The model under review builds one solid part; all positions refer to its coordinate system, in mm. Round coordinates to 2 decimals unless told otherwise and drop trailing zeros. Loops run counter-clockwise (first coordinate to the right, second up) from the corner with the lowest first, then second, coordinate; pieces in that order, holes last. Notation, with made-up numbers: (79, -13.5) - (133, -13.5) arc R31 ccw to (133, 19.5) - close; hole circle Ø2 at (52.5, -11.75). An arc over 180 degrees is marked (long way). Answer as CSV lines item,"result".
from build123d import *

# Parameters (mm, degrees)
SKETCH1_R           = 4
BOSS_EXTRUDE1_DEPTH = 50
CHAMFER1_SIZE       = 0.25
CHAMFER2_SIZE       = 0.25
CUT_EXTRUDE2_DEPTH  = 51.318982502


with BuildPart() as part:
    # Sketch1 → Boss-Extrude1 (new body)
    with BuildSketch(Plane.XY):
        Circle(SKETCH1_R)
    extrude(amount=BOSS_EXTRUDE1_DEPTH)

    # Chamfer1
    chamfer1_edges = [part.edges().sort_by_distance(p)[0] for p in [
        (-4, 0, 50),
    ]]
    chamfer(chamfer1_edges, length=CHAMFER1_SIZE)

    # Chamfer2
    chamfer2_edges = [part.edges().sort_by_distance(p)[0] for p in [
        (-4, 0, 0),
    ]]
    chamfer(chamfer2_edges, length=CHAMFER2_SIZE)

    # Sketch4 → Cut-Extrude2 (cut, through all)
    with BuildSketch(Plane.XY.offset(50)):
        with BuildLine():
            Line((-1.5, 3.708099244), (1.5, 3.708099244))
            ThreePointArc((1.5, 3.708099244), (0, 4), (-1.5, 3.708099244))
        make_face()
    extrude(amount=-CUT_EXTRUDE2_DEPTH, mode=Mode.SUBTRACT)


solid = part.part
1. Wall thickness on probe 1 along Y at (x, z) = (1.75, 31.5); probe 2 along Y at (x, z) = (1.5, 14); probe 3 along X at (y, z) = (2.75, 44): over which ranges is each line inside the solid? List them lowest first.
Numbers:
probe 1,"y = -3.6 to 3.6"
probe 2,"y = -3.71 to 3.71"
probe 3,"x = -2.9 to 2.9"
2. Draft analysis for pull direction X (two halves, no side actions). For faces 1 (the face through (0, 0, 50)), 2 (the face through (0, -4, 25)), state which applies: +X half, -X half, draft (parallel to the pull), parting line (faces both ways), or undercut.
Numbers:
face 1,"draft"
face 2,"parting line"
3. Take a section at A-A (z = 46). State the section outline as (x, y) points.
Numbers:
outline,"(-1.5, 3.71) arc R4 ccw (long way) to (1.5, 3.71) - close"
4. Clearance check with flat-ended pins moving along their axes: pin 1 (2 mm diameter, centred on x = -1.5, z = 35, fed in from -Y); pin 2 (3 mm diameter, centred on y = 2, z = 34.5, fed in from +X). State where each tip first meets the part, or that it passes through.
Numbers:
pin 1,"stops at y = -3.97"
pin 2,"stops at x = 3.97"
